Could you check a few things on this model? Use its own coordinates, in mm. Give positions to 0.01 mm unless a question says otherwise; leave off trailing zeros. Write each loop counter-clockwise with the first axis right and the second up, starting at its lowest first coordinate (ties: lowest second). Pieces come first, ordered by that corner, then holes. Notation, with made-up numbers: M -31,61.5 L -11,61.5 A10 ccw -11,79.5 Z; hole C -26.5,-6.5 d9. An arc over 180 degrees is marked long. Use one line per item in the form item = value.
from build123d import *

# Parameters (mm, degrees)
F0_R     = 36.6576669804
F0_R_2   = 32.6402559025
F0_R_3   = 8.5697598479
F0_R_4   = 8.6296556848
F0_R_5   = 8.0708127358
F0_R_6   = 7.8935022325
F0_R_7   = 8.3883706744
F1_DEPTH = 25.4
F2_DEPTH = 0.254


with BuildPart() as f1:
    # F0 (on Front) → F1 (new body)
    with BuildSketch(Plane.XZ):
        Circle(F0_R)
        Circle(F0_R_2, mode=Mode.SUBTRACT)
        Circle(F0_R_2)
        with Locations((0, -20.7587890327)):
            Circle(F0_R_3, mode=Mode.SUBTRACT)
        with Locations((-20.3415248543, 0)):
            Circle(F0_R_4, mode=Mode.SUBTRACT)
        Circle(F0_R_5, mode=Mode.SUBTRACT)
        with Locations((19.2983709276, 0)):
            Circle(F0_R_6, mode=Mode.SUBTRACT)
        with Locations((0, 18.8811086118)):
            Circle(F0_R_7, mode=Mode.SUBTRACT)
    extrude(amount=F1_DEPTH)

    # F2 (add): a face of the model
    f2_faces = [f1.faces().sort_by_distance(p)[0] for p in [
        (-9.6065952441, -25.4, -20.7587890327),
    ]]
    extrude(f2_faces, amount=F2_DEPTH)


solid = f1.part
1) I want a section at D-D, the plane x = -24.5. Please give me the cut outline in (y, z).
Checked values:
outline = M -25.65,-27.27 L 0,-27.27 L 0,-7.56 L -25.65,-7.56 Z; M -25.65,7.56 L 0,7.56 L 0,27.27 L -25.65,27.27 Z
2) I want a section at B-B, the plane x = 0. Please give me the cut outline in (y, z), plus the area to 3 significant figures.
Checked values:
outline = M -25.65,-36.66 L 0,-36.66 L 0,-29.33 L -25.65,-29.33 Z; M -25.65,-12.19 L 0,-12.19 L 0,-8.07 L -25.65,-8.07 Z; M -25.65,8.07 L 0,8.07 L 0,10.49 L -25.65,10.49 Z; M -25.65,27.27 L 0,27.27 L 0,36.66 L -25.65,36.66 Z
area = 597 mm2
3) Thinking about a two-plate mould opening in Z: for faces 1 (the cylindrical face through (-29.09, -12.647, -22.306)), 2 (the cylindrical face through (-1.116, -12.647, -12.262)), 3 (the flat face through (-1, 0, 9)), which applies, released by +Z, released by -Z, zero draft, split by the parting line, or undercut?
Checked values:
face_1 = split by the parting line
face_2 = undercut
face_3 = zero draft
4) For pin 1 Ø4 at (x, z) = (-8.5, -13) entering from +Y; pin 2 Ø12.5 at (x, z) = (19.3, 0) entering from -Y; pin 3 Ø4 at (y, z) = (-12.5, -23.5) entering from +X; pin 4 Ø2 at (y, z) = (-4, -12.5) entering from +X, each with a flat end and sliding along its axis, tell me the tip position at first contact or that it passes through.
Checked values:
pin_1 = 0
pin_2 = through
pin_3 = 29.69
pin_4 = 34.81
5) I want a section at A-A, the plane z = 0. Please give me the cut outline in (x, y).
Checked values:
outline = M -36.66,-25.65 L -28.97,-25.65 L -28.97,0 L -36.66,0 Z; M -11.71,-25.65 L -8.07,-25.65 L -8.07,0 L -11.71,0 Z; M 8.07,-25.65 L 11.4,-25.65 L 11.4,0 L 8.07,0 Z; M 27.19,-25.65 L 36.66,-25.65 L 36.66,0 L 27.19,0 Z
6) If I drill on L1, parallel to Z at x = 0, y = -13; L2, parallel to X at y = -22.5, z = -1.5; L3, parallel to Z at x = -5.5, y = -18, over which ranges is the centre line in solid material (lowest first)?
Checked values:
L1 = -36.66 to -29.33, -12.19 to -8.07, 8.07 to 10.49, 27.27 to 36.66
L2 = -36.63 to -28.84, -11.84 to -7.93, 7.93 to 11.55, 27.05 to 36.63
L3 = -36.24 to -27.33, -14.19 to -5.91, 5.91 to 12.55, 25.21 to 36.24
7) I want a section at C-C, the plane z = 22.5. Please give me the cut outline in (x, y), plus the area to 3 significant figures.
Checked values:
outline = M -28.94,-25.65 L -7.57,-25.65 L -7.57,0 L -28.94,0 Z; M 7.57,-25.65 L 28.94,-25.65 L 28.94,0 L 7.57,0 Z
area = 1,100 mm2
